```python
from build123d import *

# Parameters (mm, degrees)
SKETCH1_W           = 95.25
SKETCH1_H           = 195.2625
BOSS_EXTRUDE1_DEPTH = 12.7
FILLET1_R           = 6.35
SKETCH2_W           = 12.7
SKETCH2_H           = 6.35
CUT_EXTRUDE1_DEPTH  = 12.7


with BuildPart() as part:
    # Sketch1 → Boss-Extrude1 (new body)
    with BuildSketch(Plane(origin=(0, 0, 0), x_dir=(1, 0, 0), z_dir=(0, 1, 0))):
        with Locations((47.625, 97.63125)):
            Rectangle(SKETCH1_W, SKETCH1_H)
    extrude(amount=BOSS_EXTRUDE1_DEPTH)

    # Fillet1
    fillet1_edges = [part.edges().sort_by_distance(p)[0] for p in [
        (95.25, 12.7, -97.63125),
        (47.625, 12.7, -195.2625),
        (0, 12.7, -97.63125),
        (47.625, 0, -195.2625),
        (95.25, 0, -97.63125),
        (47.625, 0, 0),
        (0, 0, -97.63125),
        (0, 6.35, -195.2625),
        (95.25, 6.35, -195.2625),
        (95.25, 6.35, 0),
        (0, 6.35, 0),
        (47.625, 12.7, 0),
    ]]
    fillet(fillet1_edges, radius=FILLET1_R - 0.0001)  # a hair under: the kernel refuses the full size

    # Sketch2 → Cut-Extrude1 (cut)
    with BuildSketch(Plane.XY):
        with Locations((76.2, 6.35)):
            Rectangle(SKETCH2_W, SKETCH2_H)
        with Locations((60.325, 6.35)):
            Rectangle(SKETCH2_W, SKETCH2_H)
        with Locations((44.45, 6.35)):
            Rectangle(SKETCH2_W, SKETCH2_H)
    extrude(amount=-CUT_EXTRUDE1_DEPTH, mode=Mode.SUBTRACT)


solid = part.part
```
Build history of the part. All positions in model axes, mm. A direction names the side the tool comes from. Give positions to 0.01 mm unless a question says otherwise; leave off trailing zeros. One line per question, with ' | ' between items.
Q1. Tool access for faces 4 (the cylindrical face through (48.2, 10.79, -193.45)), 5 (the flat face through (76, 9.525, -7)): list every direction of +Z, -Z, +X, -X, +Y, -Y with a clear straight run to the whole face (end or side of a thin tool).
Filled sheet:
face 4: -Z, +X, -X, +Y | face 5: +Z
Q2. Drill centre lines: line 1 along X through (y, z) = (9, -12) (3 decimals); line 2 along Z through (x, y) = (51, 9.25); line 3 along X through (y, z) = (1.5, -155). Where is each one in solid material? Low to high. Write a range as [from, to].
Filled sheet:
line 1: x = [0.579, 38.1], [50.8, 53.975], [66.675, 69.85], [82.55, 94.671] | line 2: z = [-194.56, -0.7] | line 3: x = [2.25, 93]
Q3. Pull direction Y, two halves, no side cores. Call faces 1 (the cylindrical face through (48.2, 1.19, -2.65)), 2 (the cylindrical face through (1.81, 10.79, -98.91)), 3 (the flat face through (50.8, 6, -6)): pulls with the +Y half, pulls with the -Y half, needs draft (parallel to the pull), parting line crosses it, or undercut.
Filled sheet:
face 1: pulls with the -Y half | face 2: pulls with the +Y half | face 3: undercut
Q4. Drop flat-ended pins along their axis: pin 1 (3 mm diameter, centred on y = 7, z = -4, fed in from +X); pin 2 (1.5 mm diameter, centred on x = 27.5, y = 3.5, fed in from -Z); pin 3 (1.9 mm diameter, centred on x = 57.5, y = 6.5, fed in from +Z); pin 4 (3 mm diameter, centred on y = 6, z = -8, fed in from -X). Give the stop position or say it passes through.
Filled sheet:
pin 1: stops at x = 95.18 | pin 2: stops at z = -194.91 | pin 3: stops at z = -12.7 | pin 4: stops at x = 0
